from build123d import *

# Parameters (mm, degrees)
F2_DEPTH      = 25.0010001
F2_DEPTH_BACK = 25.001


with BuildPart() as f1:
    # F0 (on Front) → F1 (revolve)
    with BuildSketch(Plane.XZ):
        with BuildLine():
            Line((14, 8), (14, 0))
            Line((14, 0), (18, 0))
            Line((18, 0), (18, 2.5))
            Line((18, 2.5), (25, 2.5))
            Line((25, 2.5), (25, 5.5))
            ThreePointArc((25, 5.5), (24.4142135624, 6.9142135624), (23, 7.5))
            Line((23, 7.5), (22, 7.5))
            ThreePointArc((22, 7.5), (18.4644660941, 8.9644660941), (17, 12.5))
            Line((17, 12.5), (17, 23))
            Line((17, 23), (12, 23))
            Line((12, 23), (12, 8))
            Line((12, 8), (14, 8))
        make_face()
    revolve(axis=Axis((0, 0, 19.0387922476), (0, 0, 1)))

    # F0 (on Front) → F2 (cut, two sides)
    with BuildSketch(Plane.XZ) as f2_sk:
        Polygon((3, 23), (0, 23), (-3, 23), (-3, 18.5), (3, 18.5), align=None)
    extrude(amount=-F2_DEPTH, mode=Mode.SUBTRACT)
    extrude(f2_sk.sketch, amount=F2_DEPTH_BACK, mode=Mode.SUBTRACT)


solid = f1.part
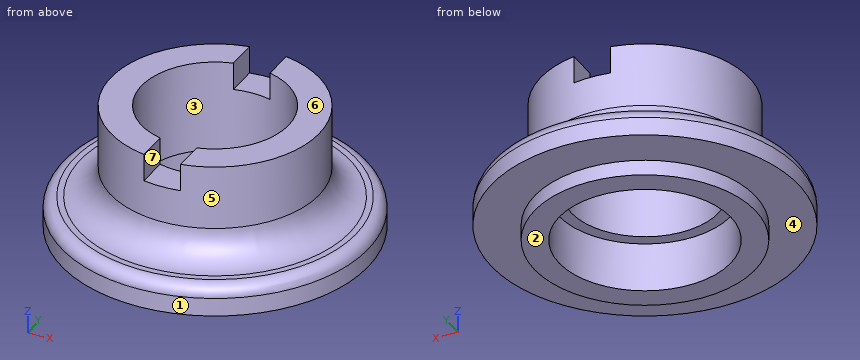
Work out the finished part from the listing and answer in its coordinate system (mm). Face numbers are marked on the shaded views. A direction names the side the tool comes from. Give positions to 0.01 mm unless a question says otherwise; leave off trailing zeros. Loops run counter-clockwise (first coordinate to the right, second up) from the corner with the lowest first, then second, coordinate; pieces in that order, holes last. Notation, with made-up numbers: M -27,13 L 22,13 A18 ccw 22,31 Z; hole C 4.25,-32 d7. An arc over 180 degrees is marked long. Use CSV: the item, a comma, the result in double quotes.
1) Find section B-B on x = 0. Write down the section's boundary in (y, z).
Answer:
outline,"M -25,2.5 L -18,2.5 L -18,0 L -14,0 L -14,8 L -12,8 L -12,18.5 L -17,18.5 L -17,12.5 A5 cw -22,7.5 L -23,7.5 A2 ccw -25,5.5 Z; M 12,8 L 14,8 L 14,0 L 18,0 L 18,2.5 L 25,2.5 L 25,5.5 A2 ccw 23,7.5 L 22,7.5 A5 cw 17,12.5 L 17,18.5 L 12,18.5 Z"
2) Consider L1, parallel to Y at x = 0, z = 15; L2, parallel to Y at x = 0, z = 3; L3, parallel to X at y = 7, z = 2.75. Determine where each line is inside the solid, lowest interval first.
Answer:
L1,"-17 to -12, 12 to 17"
L2,"-25 to -14, 14 to 25"
L3,"-24 to -12.12, 12.12 to 24"
3) Find section D-D on z = 16. Write down the section's boundary in (x, y).
Answer:
outline,"C 0,0 d34; hole C 0,0 d24"
4) Which of the six approach directions +Z, -Z, +X, -X, +Y, -Y give full straight-line access (tool end or side, diameter ignored) to the marked faces 4, 5, 6 and 7?
Answer:
face 4,"-Z"
face 5,"+Z"
face 6,"+Z, +X, -X, +Y, -Y"
face 7,"+Z, +Y, -Y"
5) Determine the mould class of the marked faces 1, 2 and 3 for opening direction Y: released by +Y, released by -Y, zero draft, split by the parting line, or undercut.
Answer:
face 1,"split by the parting line"
face 2,"zero draft"
face 3,"undercut"
6) Find section A-A on y = 0. Write down the section's boundary in (x, z).
Answer:
outline,"M -25,2.5 L -18,2.5 L -18,0 L -14,0 L -14,8 L -12,8 L -12,23 L -17,23 L -17,12.5 A5 cw -22,7.5 L -23,7.5 A2 ccw -25,5.5 Z; M 12,8 L 14,8 L 14,0 L 18,0 L 18,2.5 L 25,2.5 L 25,5.5 A2 ccw 23,7.5 L 22,7.5 A5 cw 17,12.5 L 17,23 L 12,23 Z"
7) Find section C-C on z = 20.25. Write down the section's boundary in (x, y).
Answer:
outline,"M -3,-16.73 L -3,-11.62 A12 cw -3,11.62 L -3,16.73 A17 ccw Z; M 3,-16.73 A17 ccw 3,16.73 L 3,11.62 A12 cw 3,-11.62 Z"
8) Given P1, Ø22.5, axis at x = -5.5, y = -3, coming from the -Z side; P2, Ø8, axis at y = -13.5, z = 2.5, coming from the +X side; P3, Ø5, axis at y = -13.5, z = 21, coming from the +X side; P4, Ø2, axis at x = -13, z = 8, coming from the -Y side, each flat-ended and moving along its own axis, determine where each tip first touches the part or whether it passes through.
Answer:
P1,"z = 0"
P2,"x = 23.12"
P3,"x = 12.96"
P4,"y = -20.69"
